Read the model definition and answer for the solid it produces. Units are mm, in the model's axes. A direction names the side the tool comes from. Give positions to 0.01 mm unless a question says otherwise; leave off trailing zeros. Loops run counter-clockwise (first coordinate to the right, second up) from the corner with the lowest first, then second, coordinate; pieces in that order, holes last. Notation, with made-up numbers: (29, 3) - (85, 3) arc R28 ccw to (85, 21) - close; hole circle Ø1 at (-22, -37). An arc over 180 degrees is marked (long way). Write item = value, one per line.
```python
from build123d import *

# Parameters (mm, degrees)
F1_DEPTH     = 63.5
F0_W         = 25.4
F0_H         = 19.05
F2_DEPTH     = 25.4
F3_DEPTH     = 7.9375
F5_R         = 5.08
F6_T1_DEPTH  = 17.4752
F6_T6_DEPTH  = 50.165
F6_S7_R      = 25.4
F6_T8_DEPTH  = 27
F6_T10_ANGLE = 90
F7_T1_DEPTH  = 17.4752
F7_T6_DEPTH  = 50.165
F7_S7_R      = 25.4
F7_T8_DEPTH  = 27
F7_T10_ANGLE = 90


# Not quite as in the source:
# - a fillet or chamfer that OpenCascade refuses, or shapes differently, is made with other operations: its cross-section is extruded or revolved along the edge and cut away or added


with BuildPart() as f1:
    # F0 (on Front) → F1 (new body, symmetric)
    with BuildSketch(Plane.XZ):
        Polygon((11.43, 9.525), (-30.48, 9.525), (-30.48, -9.525), (30.48, -9.525), (30.48, 9.525), align=None)
    extrude(amount=F1_DEPTH, both=True)

    # F0 (on Front) → F2 (join, symmetric)
    with BuildSketch(Plane.XZ):
        with BuildLine():
            Line((11.43, 27.0002), (11.43, 9.525))
            Line((11.43, 9.525), (30.48, 9.525))
            Line((30.48, 9.525), (30.48, 27.0002))
            ThreePointArc((30.48, 27.0002), (35.1296798487, 38.2255201513), (46.355, 42.8752))
            Line((46.355, 42.8752), (49.53, 42.8752))
            Line((49.53, 42.8752), (49.53, 61.9252))
            Line((49.53, 61.9252), (46.355, 61.9252))
            add(Edge.make_bspline(
                [(43.0102942151, 61.7646727878), (44.1205521815, 61.8325692622), (45.2356507943, 61.8861371605), (46.355, 61.9252)],
                knots=[90.4192998356, 90.4192998356, 90.4192998356, 90.4192998356, 93.0021407551, 93.0021407551, 93.0021407551, 93.0021407551], degree=3))
            ThreePointArc((43.0102942151, 61.7646727878), (20.5037962124, 50.4836172925), (11.43, 27.0002))
        make_face()
        with Locations((62.23, 52.4002)):
            Rectangle(F0_W, F0_H)
    extrude(amount=F2_DEPTH, both=True)

    # F0 (on Front) → F3 (join, symmetric)
    with BuildSketch(Plane.XZ):
        with BuildLine():
            add(Edge.make_bspline(
                [(-30.48, 9.525), (-28.7924455478, 39.4506532923), (4.142725098, 59.3877739136), (43.0102942151, 61.7646727878)],
                knots=[0, 0, 0, 0, 90.4192998356, 90.4192998356, 90.4192998356, 90.4192998356], degree=3))
            Line((-30.48, 9.525), (11.43, 9.525))
            Line((11.43, 9.525), (11.43, 27.0002))
            ThreePointArc((11.43, 27.0002), (20.5037962124, 50.4836172925), (43.0102942151, 61.7646727878))
        make_face()
    extrude(amount=F3_DEPTH, both=True)

    # F0 (on Front) → F4 (revolve)
    with BuildSketch(Plane.XZ):
        Polygon((74.93, 66.675), (74.93, 61.9252), (74.93, 42.8752), (74.93, 38.1), (100.33, 38.1), (100.33, 66.675), align=None)
    revolve(axis=Axis((74.93, 0, 52.3875), (0, 0, 1)))

    # F5
    f5_edges = [f1.edges().sort_by_distance(p)[0] for p in [
        (30.48, -63.5, 0),
        (-30.48, -63.5, 0),
        (30.48, 63.5, 0),
        (-30.48, 63.5, 0),
    ]]
    fillet(f5_edges, radius=F5_R)

    # F6: fillet of radius 5.08 on 1 edges, made by hand

    # F6_s2 → F6_t1 (cut)
    with BuildSketch(Plane.XY.offset(9.525)):
        with BuildLine():
            ThreePointArc((30.48, -20.32), (28.9921024484, -23.9121024484), (25.4, -25.4))
            Line((25.4, -25.4), (30.48, -25.4))
            Line((30.48, -25.4), (30.48, -20.32))
        make_face()
    extrude(amount=F6_T1_DEPTH, mode=Mode.SUBTRACT)


with BuildPart() as f6_tool4:
    # F6_s5 → F6_t6 (new body)
    with BuildSketch(Plane.YZ.offset(46.355)):
        with BuildLine():
            ThreePointArc((-25.4, 47.9552), (-23.9121024484, 44.3630975516), (-20.32, 42.8752))
            Line((-20.32, 42.8752), (-25.4, 42.8752))
            Line((-25.4, 42.8752), (-25.4, 47.9552))
        make_face()
    extrude(amount=F6_T6_DEPTH)

    # F6_s7 → F6_t8 (cut, symmetric)
    with BuildSketch(Plane.XY.offset(45.4)):
        with Locations((74.93, 0)):
            Circle(F6_S7_R)
    extrude(amount=F6_T8_DEPTH, both=True, mode=Mode.SUBTRACT)


with BuildPart() as f1_1:
    add(f1.part)

    # F6_t3: cut F6_tool4
    add(f6_tool4.part, mode=Mode.SUBTRACT)

    # F6_s9 → F6_t10 (revolve, cut)
    with BuildSketch(Plane.XY.offset(27.0002)):
        with BuildLine():
            ThreePointArc((30.48, -20.32), (28.9921024484, -23.9121024484), (25.4, -25.4))
            Line((25.4, -25.4), (30.48, -25.4))
            Line((30.48, -25.4), (30.48, -20.32))
        make_face()
    revolve(axis=Axis((46.355, -25.4, 27.0002), (0, 1, 0)), revolution_arc=F6_T10_ANGLE, mode=Mode.SUBTRACT)

    # F7: fillet of radius 5.08 on 3 edges, made by hand

    # F7_s2 → F7_t1 (cut)
    with BuildSketch(Plane.XY.offset(9.525)):
        with BuildLine():
            ThreePointArc((30.48, 20.32), (28.9921024484, 23.9121024484), (25.4, 25.4))
            Line((25.4, 25.4), (30.48, 25.4))
            Line((30.48, 25.4), (30.48, 20.32))
        make_face()
    extrude(amount=F7_T1_DEPTH, mode=Mode.SUBTRACT)


with BuildPart() as f7_tool4:
    # F7_s5 → F7_t6 (new body)
    with BuildSketch(Plane.YZ.offset(46.355)):
        with BuildLine():
            ThreePointArc((25.4, 47.9552), (23.9121024484, 44.3630975516), (20.32, 42.8752))
            Line((20.32, 42.8752), (25.4, 42.8752))
            Line((25.4, 42.8752), (25.4, 47.9552))
        make_face()
    extrude(amount=F7_T6_DEPTH)

    # F7_s7 → F7_t8 (cut, symmetric)
    with BuildSketch(Plane.XY.offset(45.4)):
        with Locations((74.93, 0)):
            Circle(F7_S7_R)
    extrude(amount=F7_T8_DEPTH, both=True, mode=Mode.SUBTRACT)


with BuildPart() as f1_2:
    add(f1_1.part)

    # F7_t3: cut F7_tool4
    add(f7_tool4.part, mode=Mode.SUBTRACT)

    # F7_s9 → F7_t10 (revolve, cut)
    with BuildSketch(Plane.XY.offset(27.0002)):
        with BuildLine():
            ThreePointArc((25.4, 25.4), (28.9921024484, 23.9121024484), (30.48, 20.32))
            Line((30.48, 20.32), (30.48, 25.4))
            Line((30.48, 25.4), (25.4, 25.4))
        make_face()
    revolve(axis=Axis((46.355, 25.4, 27.0002), (0, 1, 0)), revolution_arc=F7_T10_ANGLE, mode=Mode.SUBTRACT)


solid = f1_2.part
```
1) A cutting plane is placed at B-B on x = 81. Determine the outline of the cut face in (y, z) (3 decimals), then the cut area to 3 significant figures.
Output:
outline = (-24.664, 38.1) - (24.664, 38.1) - (24.664, 66.675) - (-24.664, 66.675) - close
area = 1,410 mm²
2) Each of these flat-tipped pins is pushed along its axis until it touches: P1, Ø6, axis at x = 6.5, z = 10.5, coming from the -Y side; P2, Ø14, axis at y = 19, z = 21, coming from the -X side; P3, Ø16.5, axis at x = -4.5, y = 31, coming from the +Z side (3 decimals); P4, Ø3, axis at x = 15, y = 19.5, coming from the +Z side. Where does it stop, or does it pass through?
Output:
P1 = -63.5
P2 = 11.43
P3 = 9.525
P4 = 45.12
3) A cutting plane is placed at A-A on y = -29.5. Determine the outline of the cut face in (x, z) (3 decimals).
Output:
outline = (-30.48, -9.525) - (30.48, -9.525) - (30.48, 9.525) - (-30.48, 9.525) - close
4) Find the intervals of material crossed by probe 1 along Z at (x, y) = (3, 8.5) (3 decimals); probe 2 along Y at (x, z) = (5, 23.5); probe 3 along Z at (x, y) = (55, 11) (3 decimals), in increasing order.
Output:
probe_1 = -9.525 to 9.525
probe_2 = -7.94 to 7.94
probe_3 = 38.1 to 66.675
5) A tool of negligible diameter and unlimited length cuts with its end or side. For faces 4 (the face through (11.43, -17, 18)), 5 (the face through (36, 25.4, 46)), 6 (the face through (57.267, -24.513, 45.087)), 7 (the face through (30.48, -1, 4)), 8 (the face through (49, -2, 61.925)), from which of +Z, -Z, +X, -X, +Y, -Y can it reach the whole face along a straight path? Write none if from no direction.
Output:
face_4 = +Z, -X, -Y
face_5 = +Z, +X, -X, +Y
face_6 = -Z, -Y
face_7 = -Z, +X, +Y, -Y
face_8 = +Z, -X
6) The mould has two halves that part along Z. Classify faces 1 (the face through (35.007, -0.284, 38.101)), 2 (the face through (29.031, 23.872, 18.14)), 3 (the face through (29.031, 61.972, 0.133)): pulls with the +Z half, pulls with the -Z half, needs draft (parallel to the pull), parting line crosses it, or undercut.
Output:
face_1 = pulls with the -Z half
face_2 = undercut
face_3 = needs draft
